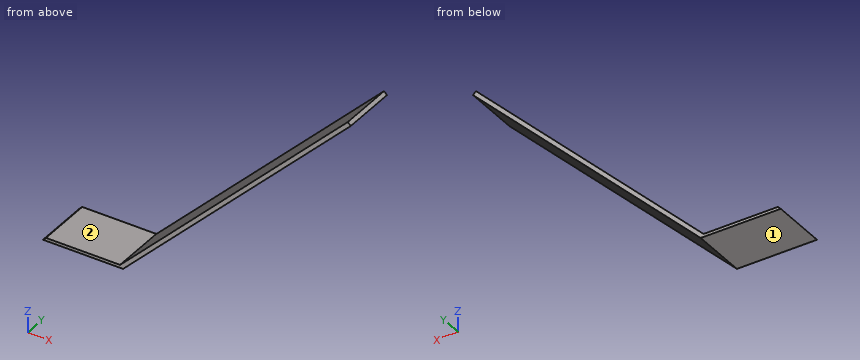
from build123d import *

# Parameters (mm, degrees)
F1_DEPTH    = 254
F2_T1_DEPTH = 332.3831903594
F3_R        = 5.08


# Not quite as in the source:
# - a fillet or chamfer that OpenCascade refuses, or shapes differently, is made with other operations: its cross-section is extruded or revolved along the edge and cut away or added


with BuildPart() as f1:
    # F0 (on Front) → F1 (new body)
    with BuildSketch(Plane.XZ):
        Polygon((1041.7304627271, 1041.6889569475), (0, 0), (-354.6740262396, 0), (-354.6520841774, -13.4706525353), (13.4701158226, -13.4706525353), (1055.2005785497, 1028.2183044122), align=None)
    extrude(amount=F1_DEPTH)

    # F2: chamfer of 15.24 on 1 edges, made by hand

    # F2_s2 → F2_t1 (cut)
    with BuildSketch(Plane.XZ.offset(-39.1915951797)):
        Polygon((-339.4340262396, 0), (-354.6492021575, -15.2399797823), (-354.6740262396, 0), align=None)
    extrude(amount=F2_T1_DEPTH, mode=Mode.SUBTRACT)

    # F3
    f3_edges = [f1.edges().sort_by_distance(p)[0] for p in [
        (0, -127, 0),
    ]]
    fillet(f3_edges, radius=F3_R)


solid = f1.part
Design review of the part built by this model. Coordinates are the model's own, in mm. Face numbers are marked on the shaded views. A direction names the side the tool comes from. Give positions to 0.01 mm unless a question says otherwise; leave off trailing zeros. Order: outer loops, then holes, each group sorted by start corner. A loop starts at its lowest first (then second) coordinate and runs counter-clockwise, first axis right, second up.
1. Add section C-C, the plane z = 132.5. State the section outline as (x, y) points, then the cut area to 3 significant figures.
Solution:
outline: (132.51, -254) - (159.45, -254) - (159.45, 0) - (132.51, 0) - close
area: 6,840 mm2
2. For pin 1 Ø10 at (x, y) = (714.5, -159) entering from -Z; pin 2 Ø5 at (y, z) = (-189, 627.5) entering from +X; pin 3 Ø6 at (x, y) = (877.5, -73.5) entering from +Z, all flat-tipped, find the tip position at first contact; note any pin that passes through.
Solution:
pin 1: stops at z = 682.53
pin 2: stops at x = 656.97
pin 3: stops at z = 880.46
3. Add section B-B, the plane x = -242. State the section outline as (y, z) points.
Solution:
outline: (-254, -13.47) - (0, -13.47) - (0, 0) - (-254, 0) - close
4. Tool access review of the marked faces 1 and 2: name each direction out of +Z, -Z, +X, -X, +Y, -Y from which nothing blocks a thin tool from reaching the whole face with its end or side.
Solution:
face 1: -Z, +X, -X, +Y, -Y
face 2: +Z, -X, +Y, -Y
5. Add section A-A, the plane y = -135.5. State the section outline as (x, z) points.
Solution:
outline: (-352.88, -13.47) - (13.47, -13.47) - (1055.2, 1028.22) - (1041.73, 1041.69) - (1.49, 1.49) arc R5.08 cw to (-2.1, 0) - (-339.43, 0) - close
6. To check wall thickness, follow L1, parallel to Z at x = -86.5, y = -106; L2, parallel to Z at x = 427.5, y = -120; L3, parallel to X at y = -238, z = 425.5. State the ranges of each line that lie inside material, in increasing order.
Solution:
L1: z = -13.47 to 0
L2: z = 400.54 to 427.48
L3: x = 425.52 to 452.46
